Work out the finished part from the listing and answer in its coordinate system (mm). A direction names the side the tool comes from. Give positions to 0.01 mm unless a question says otherwise; leave off trailing zeros. Loops run counter-clockwise (first coordinate to the right, second up) from the corner with the lowest first, then second, coordinate; pieces in that order, holes last. Notation, with made-up numbers: (-38, -33) -> (2, -33) arc R8 cw to (2, -29) -> close; hole circle Ø8 at (62.5, 9.25). An arc over 180 degrees is marked (long way). Answer as CSV lines item,"result". Start each with the question number.
1. Find the intervals of material crossed by line 1 along Y through (x, z) = (0, 17.25); line 2 along Z through (x, y) = (-4.5, 1); line 3 along X through (y, z) = (-1.5, 3.25), in increasing order.
2. Find section B-B, the plane z = 2.25. Give the vertices of the cut face in (x, y), and give its area (3 significant figures).
3. Flat-ended cylindrical pins translate along their axes: pin 1 Ø1.5 at (x, z) = (1.5, 10.5) entering from +Y; pin 2 Ø6 at (x, y) = (0, 0) entering from -Z; pin 3 Ø2 at (x, y) = (3.5, 7.5) entering from -Z; pin 4 Ø5 at (x, z) = (-3, 12) entering from -Y. Find the tip coordinate at first contact, or state that the pin passes through.
4. Find section A-A, the plane y = 0. Give the vertices of the cut face in (x, z).
5. A tool of negligible diameter and unlimited length cuts with its end or side. For faces 1 (the face through (-1.08, -4.88, 19.44)), 2 (the face through (-1.08, -4.88, 5.44)), 3 (the face through (2, -6, 25)), from which of +Z, -Z, +X, -X, +Y, -Y can it reach the whole face along a straight path? Write none if from no direction.
6. Determine the mould class of faces 4 (the face through (-2.17, -9.76, 12.34)), 5 (the face through (0, 0, 15)), 6 (the face through (2, -6, 0)) for opening direction Y: +Y half, -Y half, draft (parallel to the pull), parting line (faces both ways), or undercut.
from build123d import *

# Parameters (mm, degrees)
SKETCH_1_R      = 10
SKETCH_1_R_2    = 5
EXTRUDE_1_DEPTH = 25
FILLET_1_R      = 1
SKETCH_2_R      = 6.96901779
EXTRUDE_2_DEPTH = 5


with BuildPart() as part:
    # 草图1 → 凸台-拉伸1 (new body)
    with BuildSketch(Plane.XY):
        Circle(SKETCH_1_R)
        Circle(SKETCH_1_R_2, mode=Mode.SUBTRACT)
    extrude(amount=EXTRUDE_1_DEPTH)

    # 圆角1
    fillet_1_edges = [part.edges().sort_by_distance(p)[0] for p in [
        (-10, 0, 0),
        (-10, 0, 25),
        (-5, 0, 0),
        (-5, 0, 25),
    ]]
    fillet(fillet_1_edges, radius=FILLET_1_R)

    # 草图2 → 凸台-拉伸2 (add)
    with BuildSketch(Plane(origin=(0, 0, 10), x_dir=(-1, 0, 0), z_dir=(0, 0, -1))):
        Circle(SKETCH_2_R)
    extrude(amount=-EXTRUDE_2_DEPTH)


solid = part.part
Resolved:
1,line 1,"y = -10 to -5, 5 to 10"
1,line 2,"z = 10 to 15"
1,line 3,"x = -9.89 to -4.77, 4.77 to 9.89"
2,outline,"circle Ø20 at (0, 0); hole circle Ø10 at (0, 0)"
2,area,"236 mm^2"
3,pin 1,"stops at y = 9.97"
3,pin 2,"stops at z = 10"
3,pin 3,"stops at z = 0"
3,pin 4,"stops at y = -9.99"
4,outline,"(-10, 1) arc R1 ccw to (-9, 0) -> (-6, 0) arc R1 ccw to (-5, 1) -> (-5, 10) -> (5, 10) -> (5, 1) arc R1 ccw to (6, 0) -> (9, 0) arc R1 ccw to (10, 1) -> (10, 24) arc R1 ccw to (9, 25) -> (6, 25) arc R1 ccw to (5, 24) -> (5, 15) -> (-5, 15) -> (-5, 24) arc R1 ccw to (-6, 25) -> (-9, 25) arc R1 ccw to (-10, 24) -> close"
5,face 1,"+Z"
5,face 2,"-Z"
5,face 3,"+Z, +X, -X, +Y, -Y"
6,face 4,"parting line"
6,face 5,"undercut"
6,face 6,"draft"
